from build123d import *

# Parameters (mm, degrees)
SKETCH1_W           = 15
SKETCH1_H           = 15
SKETCH1_R           = 2.65
BOSS_EXTRUDE1_DEPTH = 3
SKETCH2_W           = 15
SKETCH2_H           = 4
BOSS_EXTRUDE2_DEPTH = 50
BOSS_EXTRUDE3_DEPTH = 3
SKETCH4_R           = 1.65
CUT_EXTRUDE1_DEPTH  = 13


with BuildPart() as part:
    # Sketch1 → Boss-Extrude1 (new body)
    with BuildSketch(Plane(origin=(0, 0, 0), x_dir=(1, 0, 0), z_dir=(0, 1, 0))):
        with Locations((7.5, 7.5)):
            Rectangle(SKETCH1_W, SKETCH1_H)
        with Locations(Location((7.5, 9, 0), (0, 0, 270))):
            Circle(SKETCH1_R, mode=Mode.SUBTRACT)
    extrude(amount=BOSS_EXTRUDE1_DEPTH)

    # Sketch2 → Boss-Extrude2 (add)
    with BuildSketch(Plane(origin=(0, 3, 0), x_dir=(1, 0, 0), z_dir=(0, 1, 0))):
        with Locations((7.5, 2)):
            Rectangle(SKETCH2_W, SKETCH2_H)
    extrude(amount=BOSS_EXTRUDE2_DEPTH)

    # Sketch3 → Boss-Extrude3 (add)
    with BuildSketch(Plane(origin=(15, 0, 0), x_dir=(0, 0, -1), z_dir=(1, 0, 0))):
        Polygon((4, 14), (15, 3), (4, 3), align=None)
    boss_extrude3 = extrude(amount=-BOSS_EXTRUDE3_DEPTH)

    # Mirror1: Boss-Extrude3 across plane
    add(boss_extrude3.mirror(Plane.ZY.offset(-7.5)))

    # Sketch4 → Cut-Extrude1 (cut)
    with BuildSketch(Plane(origin=(0, 0, -4), x_dir=(-1, 0, 0), z_dir=(0, 0, -1))):
        with Locations((-7.5, 48)):
            Circle(SKETCH4_R)
    extrude(amount=-CUT_EXTRUDE1_DEPTH, mode=Mode.SUBTRACT)


solid = part.part
Design review of the part built by this model. Coordinates are the model's own, in mm. A direction names the side the tool comes from. Coordinates: 2 decimals unless noted, no trailing zeros. Loops run counter-clockwise (first coordinate to the right, second up) from the corner with the lowest first, then second, coordinate; pieces in that order, holes last.
Item 1: Add section C-C (z = -9). Write out the cut boundary in (x, y), and give its area (3 significant figures).
Completed:
outline: (0, 0) - (4.85, 0) - (4.85, 3) - (3, 3) - (3, 9) - (0, 9) - close; (10.15, 0) - (15, 0) - (15, 9) - (12, 9) - (12, 3) - (10.15, 3) - close
area: 65.1 mm2
Item 2: For faces 4 (the flat face through (5, 3, -11)), 5 (the flat face through (1, 9, -9)), list the 3-axis set-ups (+Z, -Z, +X, -X, +Y, -Y) from which the entire face can be reached by the end or side of a thin tool; tool diameter is ignored.
Completed:
face 4: -Z, +Y
face 5: -Z, +X, -X, +Y
Item 3: Clearance check with flat-ended pins moving along their axes: pin 1 (6 mm diameter, centred on x = 5, y = 17.5, fed in from -Z); pin 2 (4.5 mm diameter, centred on x = 8, z = -9, fed in from +Y). State where each tip first meets the part, or that it passes through.
Completed:
pin 1: stops at z = -4
pin 2: stops at y = 3
Item 4: Draft analysis for pull direction Y (two halves, no side actions). For faces 1 (the flat face through (0, 18.8, -3.6)), 2 (the cylindrical face through (8.716, 49.115, -2.028)), 3 (the flat face through (7, 0, -6)), state which applies: pulls with the +Y half, pulls with the -Y half, needs draft (parallel to the pull), parting line crosses it, or undercut.
Completed:
face 1: needs draft
face 2: undercut
face 3: pulls with the -Y half
Item 5: Add section D-D (z = -12.75). Write out the cut boundary in (x, y), and give its area (3 significant figures).
Completed:
outline: (0, 0) - (15, 0) - (15, 5.25) - (12, 5.25) - (12, 3) - (3, 3) - (3, 5.25) - (0, 5.25) - close
area: 58.5 mm2
Item 6: Add section A-A (x = 7.5). Write out the cut boundary in (y, z), and give its area (3 significant figures).
Completed:
outline: (0, -15) - (3, -15) - (3, -11.65) - (0, -11.65) - close; (0, -6.35) - (3, -6.35) - (3, -4) - (46.35, -4) - (46.35, 0) - (0, 0) - close; (49.65, -4) - (53, -4) - (53, 0) - (49.65, 0) - close
area: 216 mm2
Item 7: Add section B-B (y = 48). Write out the cut boundary in (x, z).
Completed:
outline: (0, -4) - (5.85, -4) - (5.85, 0) - (0, 0) - close; (9.15, -4) - (15, -4) - (15, 0) - (9.15, 0) - close
Item 8: Wall thickness on L1, parallel to X at y = 1.15, z = -9; L2, parallel to X at y = 6.5, z = -9.75; L3, parallel to Y at x = 7.5, z = -1.7: over which ranges is each line inside the solid? List them lowest first.
Completed:
L1: x = 0 to 4.85, 10.15 to 15
L2: x = 0 to 3, 12 to 15
L3: y = 0 to 46.35, 49.65 to 53
